Here's how the part is built. I have some questions about the finished solid (model axes, mm). A direction names the side the tool comes from. Round coordinates to 2 decimals unless told otherwise and drop trailing zeros. Order: outer loops, then holes, each group sorted by start corner. A loop starts at its lowest first (then second) coordinate and runs counter-clockwise, first axis right, second up. Notation, with made-up numbers: (-37, 41.5) -> (-12, 41.5) arc R26 cw to (-12, 67.5) -> close; hole circle Ø5 at (70.5, 19.25). An arc over 180 degrees is marked (long way). Use a Markdown table: item, result. Add a question column.
from build123d import *

# Parameters (mm, degrees)
F0_R     = 9.525
F0_W     = 685.8
F0_H     = 558.2681298256
F1_DEPTH = 38.1
F2_R     = 25.4
F3_W     = 670.9210244843
F3_H     = 546.7255115509
F4_DEPTH = 71.12
F5_SIZE  = 63.5
F6_DEPTH = 21.5011


with BuildPart() as f1:
    # F0 (on Top) → F1 (new body)
    with BuildSketch(Plane.XY):
        Polygon((457.2, -381), (457.2, 381), (342.9, 381), (342.9, 279.1340649128), (342.9, -279.1340649128), (342.9, -381), align=None)
        with Locations((400.05, -330.2)):
            Circle(F0_R, mode=Mode.SUBTRACT)
        with Locations((400.05, 330.2)):
            Circle(F0_R, mode=Mode.SUBTRACT)
        Rectangle(F0_W, F0_H)
        Polygon((-342.9, -279.1340649128), (-342.9, 279.1340649128), (-342.9, 381), (-457.2, 381), (-457.2, -381), (-342.9, -381), align=None)
        with Locations((-400.05, -330.2)):
            Circle(F0_R, mode=Mode.SUBTRACT)
        with Locations((-400.05, 330.2)):
            Circle(F0_R, mode=Mode.SUBTRACT)
    extrude(amount=F1_DEPTH)

    # F2
    f2_edges = [f1.edges().sort_by_distance(p)[0] for p in [
        (-457.2, -381, 19.05),
        (-342.9, -381, 19.05),
        (342.9, -381, 19.05),
        (457.2, -381, 19.05),
        (342.9, 381, 19.05),
        (-457.2, 381, 19.05),
        (-342.9, -279.134065, 19.05),
        (342.9, -279.134065, 19.05),
        (457.2, 381, 19.05),
        (-342.9, 279.134065, 19.05),
        (-342.9, 381, 19.05),
        (342.9, 279.134065, 19.05),
    ]]
    fillet(f2_edges, radius=F2_R)

    # F3 (on face) → F4 (join)
    with BuildSketch(Plane.XY.offset(38.1)):
        Rectangle(F3_W, F3_H)
    extrude(amount=F4_DEPTH)

    # F5
    f5_edges = [f1.edges().sort_by_distance(p)[0] for p in [
        (0, 273.362756, 109.22),
        (335.460512, 0, 109.22),
        (-335.460512, 0, 109.22),
        (0, -273.362756, 109.22),
    ]]
    chamfer(f5_edges, length=F5_SIZE)

    # F6 (add): a face of the model
    f6_faces = [f1.faces().sort_by_distance(p)[0] for p in [
        (0, 0, 0),
    ]]
    extrude(f6_faces, amount=F6_DEPTH)


solid = f1.part
(1) I want a section at B-B on y = 55. List the corners of the cut face in (x, z) for me, and give its area (3 significant figures).
(2) I'm going to push flat-ended pins straight in: P1, Ø3, axis at x = -336.5, z = 43.5, coming from the +Y side; P2, Ø3, axis at x = 260.5, z = 4.5, coming from the +Y side; P3, Ø5, axis at x = -210.5, z = 28, coming from the -Y side; P4, Ø17, axis at x = 400.05, y = 330.2, coming from the +Z side. Where does each tip first touch, or does it pass through?
(3) I want a section at D-D on z = 80. List the corners of the cut face in (x, y) for me.
(4) If we mould it in two halves opening along X, with no side actions, what happens to faces 1 (the flat face through (-342.9, 330, 9)), 2 (the flat face through (-457.2, 5, 9)), 3 (the flat face through (-4, 279.134, 9)), 4 (the flat face through (400, -381, 9))? For each: pulls with the +X half, pulls with the -X half, needs draft (parallel to the pull), parting line crosses it, or undercut.
(5) Please list where these lines run through material, in increasing order: probe 1 along Y at (x, z) = (-400.05, 4) (3 decimals); probe 2 along X at (y, z) = (-156, 102); probe 3 along Z at (x, y) = (409.5, 271). Write a range as from..to.
(6) I want a section at A-A on z = 27. List the corners of the cut face in (x, y) for me (3 decimals), and give its area (3 significant figures).
(7) On a 3-axis mill with a long thin cutter (end or side, diameter ignored), from which of +Z, -Z, +X, -X, +Y, -Y can I reach the whole of each face in a straight line? I mean faces 5 (the flat face through (-400, -381, 9)), 6 (the flat face through (-4, -279.134, 9)), 7 (the cylindrical face through (-335.262, 286.377, 8.717)). Say none if no direction works.
(8) I want a section at C-C on x = -179. List the corners of the cut face in (y, z) for me.
Output:
| question | item | result |
|---|---|---|
| 1 | outline | (-457.2, -21.5) -> (457.2, -21.5) -> (457.2, 38.1) -> (335.46, 38.1) -> (335.46, 45.72) -> (271.96, 109.22) -> (-271.96, 109.22) -> (-335.46, 45.72) -> (-335.46, 38.1) -> (-457.2, 38.1) -> close |
| 1 | area | 98,200 mm² |
| 2 | P1 | y = 273.36 |
| 2 | P2 | y = 279.13 |
| 2 | P3 | y = -279.13 |
| 2 | P4 | through |
| 3 | outline | (-301.18, -239.08) -> (301.18, -239.08) -> (301.18, 239.08) -> (-301.18, 239.08) -> close |
| 4 | face 1 | undercut |
| 4 | face 2 | pulls with the -X half |
| 4 | face 3 | undercut |
| 4 | face 4 | needs draft |
| 5 | probe 1 | -381..-339.725, -320.675..320.675, 339.725..381 |
| 5 | probe 2 | -279.18..279.18 |
| 5 | probe 3 | -21.5..38.1 |
| 6 | outline | (-457.2, -355.6) arc R25.4 ccw to (-431.8, -381) -> (-368.3, -381) arc R25.4 ccw to (-342.9, -355.6) -> (-342.9, -304.534) arc R25.4 cw to (-317.5, -279.134) -> (317.5, -279.134) arc R25.4 cw to (342.9, -304.534) -> (342.9, -355.6) arc R25.4 ccw to (368.3, -381) -> (431.8, -381) arc R25.4 ccw to (457.2, -355.6) -> (457.2, 355.6) arc R25.4 ccw to (431.8, 381) -> (368.3, 381) arc R25.4 ccw to (342.9, 355.6) -> (342.9, 304.534) arc R25.4 cw to (317.5, 279.134) -> (-317.5, 279.134) arc R25.4 cw to (-342.9, 304.534) -> (-342.9, 355.6) arc R25.4 ccw to (-368.3, 381) -> (-431.8, 381) arc R25.4 ccw to (-457.2, 355.6) -> close; hole circle Ø19.05 at (-400.05, -330.2); hole circle Ø19.05 at (-400.05, 330.2); hole circle Ø19.05 at (400.05, -330.2); hole circle Ø19.05 at (400.05, 330.2) |
| 6 | area | 555,000 mm² |
| 7 | face 5 | +Z, -Z, +X, -X, -Y |
| 7 | face 6 | +Z, -Z, -Y |
| 7 | face 7 | +Z, -Z, +Y |
| 8 | outline | (-279.13, -21.5) -> (279.13, -21.5) -> (279.13, 38.1) -> (273.36, 38.1) -> (273.36, 45.72) -> (209.86, 109.22) -> (-209.86, 109.22) -> (-273.36, 45.72) -> (-273.36, 38.1) -> (-279.13, 38.1) -> close |
